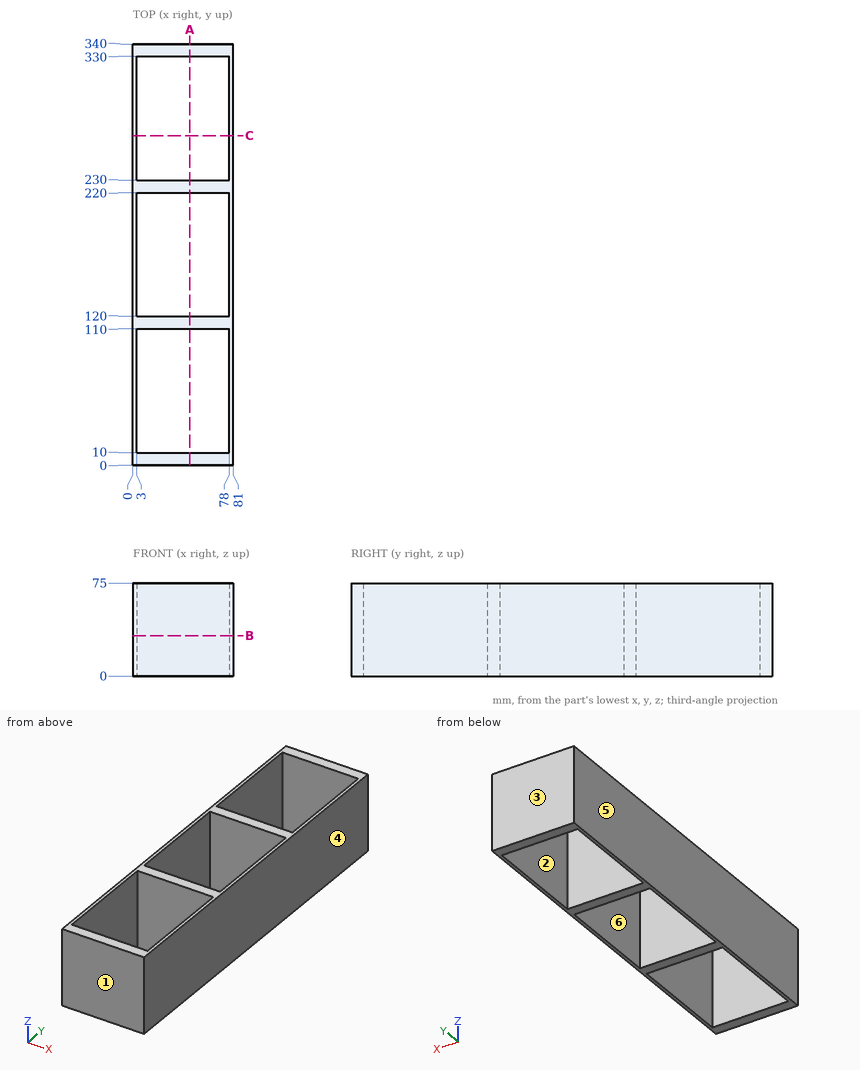
Input: dimensioned drawing with shaded views. Units: mm. Origin: part minimum x, y, z. A direction names the side the tool comes from. Coordinates: 2 decimals unless noted, no trailing zeros. Order: outer loops, then holes, each group sorted by start corner. A loop starts at its lowest first (then second) coordinate and runs counter-clockwise, first axis right, second up. Notation, with made-up numbers: M 34.5,36.25 L 61.5,36.25 A19 cw 61.5,41.25 Z; hole C 57.25,79.5 d8. An arc over 180 degrees is marked long. Write each question's results on one line, items separated by ' | '. Start each with the question number.
Item 1: Cut plane C-C (y = 266). Return loops of the section in (x, z).
Item 2: Draft query along Y for the marked faces 1, 2, 3 and 4. Return one class per face: pulls with the +Y half, pulls with the -Y half, needs draft (parallel to the pull), parting line crosses it, or undercut.
Item 3: Set-up query: the marked faces 5 and 6. Return all of +Z, -Z, +X, -X, +Y, -Y with unobstructed straight access to the full face (end or side cutting, diameter ignored); none if empty.
Item 4: Cut plane B-B (z = 32.5). Return loops of the section in (x, y).
Item 5: Cut plane A-A (x = 46). Return loops of the section in (y, z), and give its area (3 significant figures).
Item 6: Line query: probe 1 along Y at (x, z) = (30.5, 16.5); probe 2 along X at (y, z) = (99, 32). Output: solid intervals per line, ascending.
Item 7: First-contact query: pin 1 Ø22.5 at (y, z) = (291, 49) entering from -X. Flat tip, straight axial feed; report the tip coordinate or a pass-through.
Checked values:
1) outline: M 0,0 L 3,0 L 3,75 L 0,75 Z; M 78,0 L 81,0 L 81,75 L 78,75 Z
2) face 1: pulls with the -Y half | face 2: undercut | face 3: pulls with the +Y half | face 4: needs draft
3) face 5: +Z, -Z, -X, +Y, -Y | face 6: +Z, -Z
4) outline: M 0,0 L 81,0 L 81,340 L 0,340 Z; hole M 3,10 L 78,10 L 78,110 L 3,110 Z; hole M 3,120 L 78,120 L 78,220 L 3,220 Z; hole M 3,230 L 78,230 L 78,330 L 3,330 Z
5) outline: M 0,0 L 10,0 L 10,75 L 0,75 Z; M 110,0 L 120,0 L 120,75 L 110,75 Z; M 220,0 L 230,0 L 230,75 L 220,75 Z; M 330,0 L 340,0 L 340,75 L 330,75 Z | area: 3,000 mm2
6) probe 1: y = 0 to 10, 110 to 120, 220 to 230, 330 to 340 | probe 2: x = 0 to 3, 78 to 81
7) pin 1: stops at x = 0
